Work out the finished part from the listing and answer in its coordinate system (mm). A direction names the side the tool comes from. Coordinates: 2 decimals unless noted, no trailing zeros. Write each loop counter-clockwise with the first axis right and the second up, starting at its lowest first coordinate (ties: lowest second). Pieces come first, ordered by that corner, then holes. Notation, with made-up numbers: (80.5, 86.25) - (137.5, 86.25) arc R17 cw to (137.5, 101.25) - close; hole circle Ø4 at (20, 28.5). An arc over 180 degrees is marked (long way). One line per item, written item: value.
```python
from build123d import *

# Parameters (mm, degrees)
F1_DEPTH = 100
F3_DEPTH = 25
F4_W     = 12.3
F4_H     = 8.3
F5_DEPTH = 25


with BuildPart() as f1:
    # F0 (on Front) → F1 (new body)
    with BuildSketch(Plane.XZ):
        Polygon((-16.789507, 0), (0, 0), (0, 12), (8, 20), (8, 22), (-5.789507, 22), (-16.789507, 11), align=None)
    extrude(amount=F1_DEPTH)

    # F2 (on face) → F3 (cut)
    with BuildSketch(Plane.YZ):
        with BuildLine():
            Line((-74.858745, 6.3), (-85.141255, 6.3))
            ThreePointArc((-85.141255, 6.3), (-80, 0.85), (-74.858745, 6.3))
        make_face()
        with BuildLine():
            Line((-24.858745, 6.3), (-35.141255, 6.3))
            ThreePointArc((-35.141255, 6.3), (-30, 0.85), (-24.858745, 6.3))
        make_face()
    extrude(amount=-F3_DEPTH, mode=Mode.SUBTRACT)

    # F4 (on face) → F5 (cut)
    with BuildSketch(Plane.YZ.offset(8)):
        with Locations((-9, 13)):
            Rectangle(F4_W, F4_H)
    extrude(amount=-F5_DEPTH, mode=Mode.SUBTRACT)


solid = f1.part
```
Item 1: Section C-C, the plane y = -39 is taken. Determine the outline of the cut face in (x, z), then the cut area to 3 significant figures.
Evaluation:
outline: (-16.79, 0) - (0, 0) - (0, 12) - (8, 20) - (8, 22) - (-5.79, 22) - (-16.79, 11) - close
area: 357 mm2
Item 2: Given pin 1 (6 mm diameter, centred on x = -9.5, y = -69, fed in from +Z); pin 2 (6 mm diameter, centred on y = -55.5, z = 15, fed in from -X); pin 3 (3.5 mm diameter, centred on y = -48.5, z = 4.5, fed in from +X); pin 4 (2 mm diameter, centred on y = -77.5, z = 4.5, fed in from +X), each flat-ended and moving along its own axis, determine where each tip first touches the part or whether it passes through.
Evaluation:
pin 1: stops at z = 21.29
pin 2: stops at x = -15.79
pin 3: stops at x = 0
pin 4: passes through
Item 3: Consider probe 1 along Y at (x, z) = (-12, 11.25); probe 2 along Y at (x, z) = (-0.25, 5); probe 3 along X at (y, z) = (-64, 5.75). Determine where each line is inside the solid, lowest interval first.
Evaluation:
probe 1: y = -100 to -15.15, -2.85 to 0
probe 2: y = -100 to -85.05, -74.95 to -35.05, -24.95 to 0
probe 3: x = -16.79 to 0
Item 4: Section A-A, the plane y = -80 is taken. Determine the outline of the cut face in (x, z).
Evaluation:
outline: (-16.79, 0) - (0, 0) - (0, 0.85) - (-16.79, 0.85) - close; (-16.79, 6.3) - (0, 6.3) - (0, 12) - (8, 20) - (8, 22) - (-5.79, 22) - (-16.79, 11) - close
Item 5: Section B-B, the plane z = 4 is taken. Determine the outline of the cut face in (x, y), then the cut area to 3 significant figures.
Evaluation:
outline: (-16.79, -100) - (0, -100) - (0, -84.75) - (-16.79, -84.75) - close; (-16.79, -75.25) - (0, -75.25) - (0, -34.75) - (-16.79, -34.75) - close; (-16.79, -25.25) - (0, -25.25) - (0, 0) - (-16.79, 0) - close
area: 1,360 mm2
Item 6: Determine the mould class of faces 1 (the face through (-8.28, -80.12, 0.85)), 2 (the face through (-5, 0, 11)), 3 (the face through (-9, -49, 0)) for opening direction Y: +Y half, -Y half, draft (parallel to the pull), parting line (faces both ways), or undercut.
Evaluation:
face 1: undercut
face 2: +Y half
face 3: draft
Item 7: Section D-D, the plane x = -8.75 is taken. Determine the outline of the cut face in (y, z).
Evaluation:
outline: (-100, 0) - (0, 0) - (0, 19.04) - (-100, 19.04) - close; hole (-85.14, 6.3) arc R5.15 ccw (long way) to (-74.86, 6.3) - close; hole (-35.14, 6.3) arc R5.15 ccw (long way) to (-24.86, 6.3) - close; hole (-15.15, 8.85) - (-2.85, 8.85) - (-2.85, 17.15) - (-15.15, 17.15) - close
Item 8: Which of the six approach directions +Z, -Z, +X, -X, +Y, -Y give full straight-line access (tool end or side, diameter ignored) to faces 4 (the face through (0, -49, 6)), 5 (the face through (-5, -100, 11)), 6 (the face through (-6, -15.15, 13))?
Evaluation:
face 4: -Z, +X, +Y, -Y
face 5: +Z, -Z, +X, -X, -Y
face 6: +X, -X
